```python
from build123d import *

# Parameters (mm, degrees)
PAD003_DEPTH    = 3.3
SKETCH016_R     = 4
POCKET005_DEPTH = 5
SKETCH007_W     = 11
SKETCH007_H     = 18
POCKET006_DEPTH = 2.7
SKETCH008_W     = 5.388972
SKETCH008_H     = 3.069046
POCKET007_DEPTH = 1
SKETCH018_R     = 2
POCKET008_DEPTH = 5
POCKET009_DEPTH = 0.85
SKETCH020_W     = 0.35
SKETCH020_H     = 0.6
POCKET010_DEPTH = 25
FILLET_R        = 1
SKETCH034_W     = 5
SKETCH034_H     = 1
POCKET020_DEPTH = 0.35
SKETCH035_W     = 5
SKETCH035_H     = 1
POCKET021_DEPTH = 0.35


with BuildPart() as part:
    # Sketch005 → Pad003 (new body)
    with BuildSketch(Plane.XY):
        with BuildLine():
            Line((-10.15, 18.375), (10.15, 18.375))
            Line((10.15, 18.375), (10.15, -17.75))
            Line((3.33, -24.57), (10.15, -17.75))
            ThreePointArc((-3.33, -24.57), (0, -26.037308), (3.33, -24.57))
            Line((-10.15, -17.75), (-3.33, -24.57))
            Line((-10.15, -17.75), (-10.15, 18.375))
        make_face()
    extrude(amount=PAD003_DEPTH)

    # Sketch016 → Pocket005 (cut)
    with BuildSketch(Plane.XY):
        with Locations((0, 10.2)):
            Circle(SKETCH016_R)
    extrude(amount=POCKET005_DEPTH, mode=Mode.SUBTRACT)

    # Sketch007 (on Face4 of Pocket005) → Pocket006 (cut)
    with BuildSketch(Plane(origin=(0, 0, 0), x_dir=(1, 0, 0), z_dir=(0, 0, -1))):
        with Locations((0, 5.277613)):
            Rectangle(SKETCH007_W, SKETCH007_H)
    extrude(amount=-POCKET006_DEPTH, mode=Mode.SUBTRACT)

    # Sketch008 → Pocket007 (cut)
    with BuildSketch(Plane.XY):
        with Locations((-2.024069, -8.897589)):
            Rectangle(SKETCH008_W, SKETCH008_H)
    extrude(amount=POCKET007_DEPTH, mode=Mode.SUBTRACT)

    # Sketch018 → Pocket008 (cut)
    with BuildSketch(Plane.XY):
        with Locations((0, -21.525)):
            Circle(SKETCH018_R)
    extrude(amount=POCKET008_DEPTH, mode=Mode.SUBTRACT)

    # Sketch019 → Pocket009 (cut)
    with BuildSketch(Plane.XY):
        with BuildLine():
            Line((-9.35, 17.285263), (-9.35, -17.814737))
            Line((-9.35, -17.814737), (-2.6, -24.564737))
            ThreePointArc((-2.6, -24.564737), (0, -25.525), (2.6, -24.564737))
            Line((2.6, -24.564737), (9.35, -17.814737))
            Line((9.35, -17.814737), (9.35, 17.285263))
            ThreePointArc((9.35, 17.285263), (9.155303, 17.755303), (8.685263, 17.95))
            Line((8.685263, 17.95), (-8.685263, 17.95))
            ThreePointArc((-8.685263, 17.95), (-9.155303, 17.755303), (-9.35, 17.285263))
        make_face()
    extrude(amount=POCKET009_DEPTH, mode=Mode.SUBTRACT)

    # Sketch020 (on Face16 of Pocket009) → Pocket010 (cut)
    with BuildSketch(Plane.YZ.offset(-9.35)):
        with Locations((-9.625, -1.8)):
            Rectangle(SKETCH020_W, SKETCH020_H)
        with Locations((9.625, -1.8)):
            Rectangle(SKETCH020_W, SKETCH020_H)
    extrude(amount=-POCKET010_DEPTH, mode=Mode.SUBTRACT)

    # Fillet
    fillet_edges = [part.edges().sort_by_distance(p)[0] for p in [
        (10.15, -17.75, 1.65),
        (10.15, 18.375, 1.65),
        (-6.74, -21.16, 3.3),
        (-10.15, 0.3125, 3.3),
        (0, -26.037308, 3.3),
        (0, 18.375, 3.3),
        (6.74, -21.16, 3.3),
        (10.15, 0.3125, 3.3),
        (-2, -21.525, 3.3),
        (-4, 10.2, 3.3),
        (-10.15, 18.375, 1.65),
        (-10.15, -17.75, 1.65),
    ]]
    fillet(fillet_edges, radius=FILLET_R)

    # Sketch034 (on Face10 of Fillet) → Pocket020 (cut)
    with BuildSketch(Plane(origin=(-10.15, 0, 0), x_dir=(0, -1, 0), z_dir=(-1, 0, 0))):
        with Locations((0, 0.5)):
            Rectangle(SKETCH034_W, SKETCH034_H)
    extrude(amount=-POCKET020_DEPTH, mode=Mode.SUBTRACT)

    # Sketch035 (on Face11 of Pocket020) → Pocket021 (cut)
    with BuildSketch(Plane.YZ.offset(10.15)):
        with Locations((0, 0.5)):
            Rectangle(SKETCH035_W, SKETCH035_H)
    extrude(amount=-POCKET021_DEPTH, mode=Mode.SUBTRACT)


solid = part.part
```
Here's how the part is built. I have some questions about the finished solid (model axes, mm). A direction names the side the tool comes from. Give positions to 0.01 mm unless a question says otherwise; leave off trailing zeros. Order: outer loops, then holes, each group sorted by start corner. A loop starts at its lowest first (then second) coordinate and runs counter-clockwise, first axis right, second up. Notation, with made-up numbers: (7, -23) -> (56, -23) arc R13 cw to (56, -4) -> close; hole circle Ø3 at (4.25, 38.25). An arc over 180 degrees is marked (long way). Use CSV: the item, a comma, the result in double quotes. Start each with the question number.
Item 1: Suppose I cut it at D-D (y = -2). List the corners of the cut face in (x, z) for me.
Item 2: Thinking about a two-plate mould opening in Y: for faces 1 (the flat face through (0, 3.722, 2)), 2 (the flat face through (-10.15, -0.2, 1.4)), 3 (the cylindrical face through (-9.85, 18.09, 1.17)), 4 (the cylindrical face through (-0.052, -26.037, 1.134)), which applies, pulls with the +Y half, pulls with the -Y half, needs draft (parallel to the pull), parting line crosses it, or undercut?
Item 3: Suppose I cut it at A-A (x = 0). List the corners of the cut face in (y, z) for me (3 decimals), and give its area (3 significant figures).
Item 4: If I drill on probe 1 along Y at (x, z) = (0, 1.5) (3 decimals); probe 2 along X at (y, z) = (-4, 2); probe 3 along Y at (x, z) = (0.5, 0.9) (1 decimal), over which ranges is the centre line in solid material (lowest first)? Write a range as [from, to].
Item 5: Suppose I cut it at B-B (y = 10.2). List the corners of the cut face in (x, z) for me.
Item 6: Suppose I cut it at C-C (z = 1.9). List the corners of the cut face in (x, y) for me (3 decimals), and give its area (3 significant figures).
Item 7: I'm going to push flat-ended pins straight in: P1, Ø0.9, axis at x = -1.5, z = 0.5, coming from the -Y side; P2, Ø4.5, axis at x = 0, y = -21.525, coming from the -Z side; P3, Ø9, axis at x = 0.5, y = -1, coming from the -Z side. Where does each tip first touch, or does it pass through?
Item 8: On a 3-axis mill with a long thin cutter (end or side, diameter ignored), from which of +Z, -Z, +X, -X, +Y, -Y can I reach the whole of each face in a straight line? I mean faces 5 (the cylindrical face through (0.13, 18.09, 3)), 6 (the flat face through (0.1, 17.95, 0.4)), 7 (the flat face through (9.8, 0, 0.5)). Say none if no direction works.
Answer block:
1,outline,"(-10.15, 1) -> (-9.8, 1) -> (-9.8, 0) -> (-9.35, 0) -> (-9.35, 0.85) -> (-5.5, 0.85) -> (-5.5, 2.7) -> (5.5, 2.7) -> (5.5, 0.85) -> (9.35, 0.85) -> (9.35, 0) -> (9.8, 0) -> (9.8, 1) -> (10.15, 1) -> (10.15, 2.3) arc R1 ccw to (9.15, 3.3) -> (-9.15, 3.3) arc R1 ccw to (-10.15, 2.3) -> close"
2,face 1,"undercut"
2,face 2,"needs draft"
2,face 3,"pulls with the +Y half"
2,face 4,"pulls with the -Y half"
3,outline,"(-26.037, 0) -> (-25.525, 0) -> (-25.525, 0.85) -> (-23.525, 0.85) -> (-23.525, 2.3) arc R1 ccw to (-24.525, 3.3) -> (-25.037, 3.3) arc R1 ccw to (-26.037, 2.3) -> close; (-19.525, 0.85) -> (-14.278, 0.85) -> (-14.278, 2.7) -> (3.722, 2.7) -> (3.722, 0.85) -> (6.2, 0.85) -> (6.2, 2.3) arc R1 ccw to (5.2, 3.3) -> (-18.525, 3.3) arc R1 ccw to (-19.525, 2.3) -> close; (14.2, 0.85) -> (17.95, 0.85) -> (17.95, 0) -> (18.375, 0) -> (18.375, 2.3) arc R1 ccw to (17.375, 3.3) -> (15.2, 3.3) arc R1 ccw to (14.2, 2.3) -> close"
3,area,"45.6 mm^2"
4,probe 1,"y = [-26.037, -23.525], [-19.525, -14.278], [3.722, 6.2], [14.2, 18.375]"
4,probe 2,"x = [-10.15, -5.5], [5.5, 10.15]"
4,probe 3,"y = [-26, -23.5], [-19.6, -14.3], [3.7, 6.2], [14.2, 18.4]"
5,outline,"(-10.15, 0) -> (-9.35, 0) -> (-9.35, 0.85) -> (-4, 0.85) -> (-4, 2.3) arc R1 ccw to (-5, 3.3) -> (-9.15, 3.3) arc R1 ccw to (-10.15, 2.3) -> close; (4, 0.85) -> (9.35, 0.85) -> (9.35, 0) -> (10.15, 0) -> (10.15, 2.3) arc R1 ccw to (9.15, 3.3) -> (5, 3.3) arc R1 ccw to (4, 2.3) -> close"
6,outline,"(-10.15, -17.336) arc R1 ccw to (-9.857, -18.043) -> (-3.33, -24.57) arc R4.512 ccw to (3.33, -24.57) -> (9.857, -18.043) arc R1 ccw to (10.15, -17.336) -> (10.15, 17.375) arc R1 ccw to (9.15, 18.375) -> (-9.15, 18.375) arc R1 ccw to (-10.15, 17.375) -> close; hole (-5.5, -14.278) -> (5.5, -14.278) -> (5.5, 3.722) -> (-5.5, 3.722) -> close; hole circle Ø8 at (0, 10.2); hole circle Ø4 at (0, -21.525)"
6,area,"571 mm^2"
7,P1,"stops at y = -25.91"
7,P2,"stops at z = 0.85"
7,P3,"stops at z = 2.7"
8,face 5,"+Z, +X, -X, +Y"
8,face 6,"-Z"
8,face 7,"-Z, +X"
